CAD build for the part. Positions are in the model's coordinates, mm. Face numbers are marked on the shaded views. A direction names the side the tool comes from. Give positions to 0.01 mm unless a question says otherwise; leave off trailing zeros. Order: outer loops, then holes, each group sorted by start corner. A loop starts at its lowest first (then second) coordinate and runs counter-clockwise, first axis right, second up.
Item 1: Band-saw the part on A-A on y = -9.5. Give the cut face in (x, z).
Item 2: Which spindle directions (+Z, -Z, +X, -X, +Y, -Y) get a long thin tool onto all of the face, cutting with end or side? Do the marked faces 1 and 2. Say none if no direction does.
Item 3: Flat gauge pin, fed straight in: P1, Ø6.5, axis at x = 30, y = -14.5, coming from the +Z side. Where does the tip first touch, or does it go through?
Item 4: Band-saw the part on B-B on x = 30. Give the cut face in (y, z).
Item 5: Band-saw the part on C-C on z = 16.5. Give the cut face in (x, y), plus the area to 3 significant figures.
Item 6: Wall check: L1, parallel to Z at x = 29, y = -9.25; L2, parallel to X at y = -23.75, z = 15; L3, parallel to X at y = -6.25, z = 18.5. Give the ranges that are in metal, low to high.
```python
from build123d import *

# Parameters (mm, degrees)
F0_W     = 38.1
F0_H     = 31.75
F1_DEPTH = 25.4
F2_W     = 25.4
F2_H     = 19.05
F4_DEPTH = 12.7
F6_DEPTH = 25.401


with BuildPart() as f1:
    # F0 (on Front) → F1 (new body)
    with BuildSketch(Plane.XZ):
        with Locations((19.05, 15.875)):
            Rectangle(F0_W, F0_H)
    extrude(amount=F1_DEPTH)

    # F2 (on face) → F4 (cut)
    with BuildSketch(Plane.YZ.offset(38.1)):
        with Locations((-12.7, 22.225)):
            Rectangle(F2_W, F2_H)
    extrude(amount=-F4_DEPTH, mode=Mode.SUBTRACT)

    # F5 (on face) → F6 (cut, through all)
    with BuildSketch(Plane.XZ.offset(25.4)):
        Polygon((12.925296, 31.75), (25.609119, 12.724266), (25.609119, 31.75), align=None)
    extrude(amount=-F6_DEPTH, mode=Mode.SUBTRACT)


solid = f1.part
```
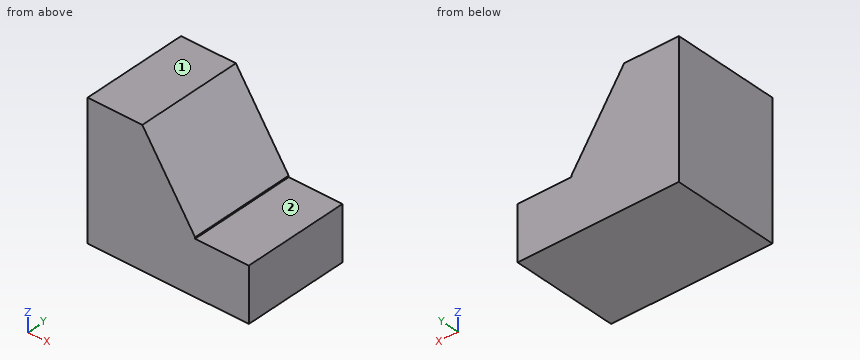
The answers:
1. outline: (0, 0) - (38.1, 0) - (38.1, 12.7) - (25.4, 12.7) - (25.4, 13.04) - (12.93, 31.75) - (0, 31.75) - close
2. face 1: +Z, +X, -X, +Y, -Y
2. face 2: +Z, +X, +Y, -Y
3. P1: stops at z = 12.7
4. outline: (-25.4, 0) - (0, 0) - (0, 12.7) - (-25.4, 12.7) - close
5. outline: (0, -25.4) - (23.09, -25.4) - (23.09, 0) - (0, 0) - close
5. area: 587 mm2
6. L1: z = 0 to 12.7
6. L2: x = 0 to 24.09
6. L3: x = 0 to 21.76
